Build history of the part. All positions in model axes, mm. Face numbers are marked on the shaded views. A direction names the side the tool comes from. Coordinates: 2 decimals unless noted, no trailing zeros. Loops run counter-clockwise (first coordinate to the right, second up) from the corner with the lowest first, then second, coordinate; pieces in that order, holes last.
Item 1: Mould opens along Y. For the marked faces 1, 2, 3 and 4 say: released by +Y, released by -Y, zero draft, split by the parting line, or undercut.
Item 2: 3-axis set-ups, long thin cutter, end or side, ignore diameter. For the marked faces 5 and 6: which of +Z, -Z, +X, -X, +Y, -Y reach the whole face in a straight line?
Item 3: Drill centre lines: line 1 along Z through (x, y) = (0, 63.7) (3 decimals); line 2 along X through (y, z) = (36.5, 3.75). Where is each one in solid material? Low to high.
Item 4: Cut at A-A (y = 52). List the corners of the cut face in (x, z) (3 decimals), and give its area (3 significant figures).
Item 5: Cut at B-B (z = 0). List the corners of the cut face in (x, y), and give its area (3 significant figures).
Item 6: Flat gauge pins, fed straight in: pin 1 (3.5 mm diameter, centred on x = 0.5, z = 0.5, fed in from -Y); pin 2 (2 mm diameter, centred on x = 0, z = 0, fed in from +Y); pin 3 (1 mm diameter, centred on x = 5, z = 1.5, fed in from -Y); pin 4 (7.5 mm diameter, centred on x = -3, y = 6, fed in from -Z) (3 decimals). Where does each tip first touch, or does it go through?
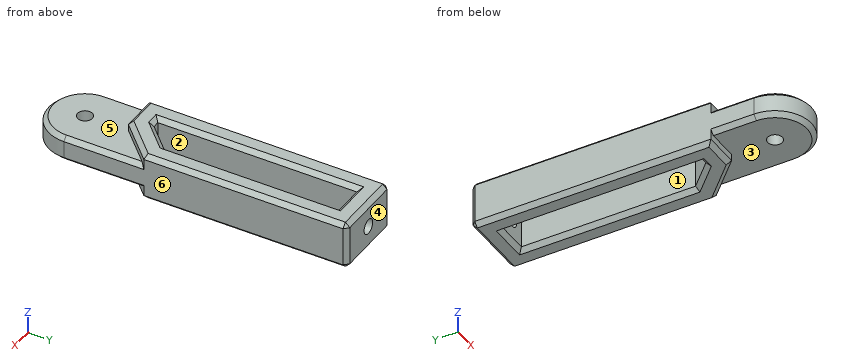
from build123d import *

# Parameters (mm, degrees)
BOSS_EXTRUDE1_DEPTH = 2.975
BOSS_EXTRUDE2_DEPTH = 2.5
BOSS_EXTRUDE3_START = -5.95
BOSS_EXTRUDE3_DEPTH = 2.5
CUT_EXTRUDE3_DEPTH  = 11.95
SKETCH6_R           = 1.7
CUT_EXTRUDE4_DEPTH  = 5.75
SKETCH7_R           = 1.7
CUT_EXTRUDE5_DEPTH  = 9.45
CHAMFER1_SIZE       = 1


with BuildPart() as part:
    # Sketch1 → Boss-Extrude1 (new body, symmetric)
    with BuildSketch(Plane.XY):
        with BuildLine():
            Line((-8.35, 0), (-8.35, 65.15))
            Line((-8.35, 65.15), (8.35, 65.15))
            Line((8.35, 65.15), (8.35, 0))
            ThreePointArc((8.35, 0), (0, -8.35), (-8.35, 0))
        make_face()
    extrude(amount=BOSS_EXTRUDE1_DEPTH, both=True)

    # Sketch4 → Boss-Extrude2 (add)
    with BuildSketch(Plane.XY.offset(2.975)):
        Polygon((-8.35, 65.15), (-8.35, 9.9), (-0.135281374, 9.9), (8.35, 18.385281374), (8.35, 65.15), align=None)
    extrude(amount=BOSS_EXTRUDE2_DEPTH)

    # Sketch4<2> → Boss-Extrude3 (add)
    with BuildSketch(Plane.XY.offset(2.975).offset(BOSS_EXTRUDE3_START)):
        Polygon((-8.35, 65.15), (-8.35, 9.9), (-0.135281374, 9.9), (8.35, 18.385281374), (8.35, 65.15), align=None)
    extrude(amount=-BOSS_EXTRUDE3_DEPTH)

    # Sketch5 → Cut-Extrude3 (cut, through all)
    with BuildSketch(Plane.XY.offset(5.475)):
        Polygon((-3.6, 14.65), (-2.102795796, 14.65), (3.6, 20.352795796), (3.6, 60.4), (-3.6, 60.4), align=None)
    extrude(amount=-CUT_EXTRUDE3_DEPTH, mode=Mode.SUBTRACT)

    # Sketch6 → Cut-Extrude4 (cut, through all)
    with BuildSketch(Plane.XZ.offset(-60.4)):
        Circle(SKETCH6_R)
    extrude(amount=-CUT_EXTRUDE4_DEPTH, mode=Mode.SUBTRACT)

    # Sketch7 → Cut-Extrude5 (cut, through all)
    with BuildSketch(Plane.XY.offset(2.975)):
        Circle(SKETCH7_R)
    extrude(amount=-CUT_EXTRUDE5_DEPTH, mode=Mode.SUBTRACT)

    # Chamfer1
    chamfer1_edges = [part.edges().sort_by_distance(p)[0] for p in [
        (-8.35, 4.95, 2.975),
        (0, 65.15, 5.475),
        (-8.35, 37.525, 5.475),
        (-4.242640687, 9.9, 5.475),
        (4.107359313, 14.142640687, 5.475),
        (8.35, 41.767640687, 5.475),
        (-8.35, 4.95, -2.975),
        (4.107359313, 14.142640687, -5.475),
        (-4.242640687, 9.9, -5.475),
        (-8.35, 37.525, -5.475),
        (0, 65.15, -5.475),
        (8.35, 41.767640687, -5.475),
        (0, -8.35, 2.975),
        (3.6, 40.376397898, -5.475),
        (0.748602102, 17.501397898, -5.475),
        (-2.851397898, 14.65, -5.475),
        (-3.6, 37.525, -5.475),
        (0, 60.4, -5.475),
        (3.6, 40.376397898, 5.475),
        (0, 60.4, 5.475),
        (-3.6, 37.525, 5.475),
        (-2.851397898, 14.65, 5.475),
        (0.748602102, 17.501397898, 5.475),
        (8.35, 9.192640687, -2.975),
        (0, -8.35, -2.975),
        (-8.35, 65.15, 0),
        (8.35, 65.15, 0),
        (8.35, 9.192640687, 2.975),
    ]]
    chamfer(chamfer1_edges, length=CHAMFER1_SIZE)


solid = part.part
Filled sheet:
1. face 1: undercut
1. face 2: undercut
1. face 3: zero draft
1. face 4: released by +Y
2. face 5: +Z, +X, -Y
2. face 6: +Z, -Z, +X, +Y, -Y
3. line 1: z = -5.475 to -1.7, 1.7 to 5.475
3. line 2: x = -8.35 to -3.6, 3.6 to 8.35
4. outline: (-8.35, -4.475) - (-7.35, -5.475) - (-4.6, -5.475) - (-3.6, -4.475) - (-3.6, 4.475) - (-4.6, 5.475) - (-7.35, 5.475) - (-8.35, 4.475) - close; (3.6, -4.475) - (4.6, -5.475) - (7.35, -5.475) - (8.35, -4.475) - (8.35, 4.475) - (7.35, 5.475) - (4.6, 5.475) - (3.6, 4.475) - close
4. area: 100 mm2
5. outline: (-8.35, 0) arc R8.35 ccw to (8.35, 0) - (8.35, 64.15) - (7.35, 65.15) - (1.7, 65.15) - (1.7, 60.4) - (3.6, 60.4) - (3.6, 20.35) - (-2.1, 14.65) - (-3.6, 14.65) - (-3.6, 60.4) - (-1.7, 60.4) - (-1.7, 65.15) - (-7.35, 65.15) - (-8.35, 64.15) - close; hole circle Ø3.4 at (0, 0)
5. area: 858 mm2
6. pin 1: stops at y = -8.35
6. pin 2: stops at y = 17.75
6. pin 3: stops at y = -7.03
6. pin 4: stops at z = -2.975
